Build history of the part. All positions in model axes, mm. Face numbers are marked on the shaded views. A direction names the side the tool comes from. Round coordinates to 2 decimals unless told otherwise and drop trailing zeros. Write each loop counter-clockwise with the first axis right and the second up, starting at its lowest first coordinate (ties: lowest second). Pieces come first, ordered by that corner, then holes. Notation, with made-up numbers: (34.25, 61.5) -> (45.25, 61.5) arc R19 ccw to (45.25, 95.5) -> close; hole circle Ø4 at (-13, -39.75). An arc over 180 degrees is marked (long way). One line per question, with ' | ' between items.
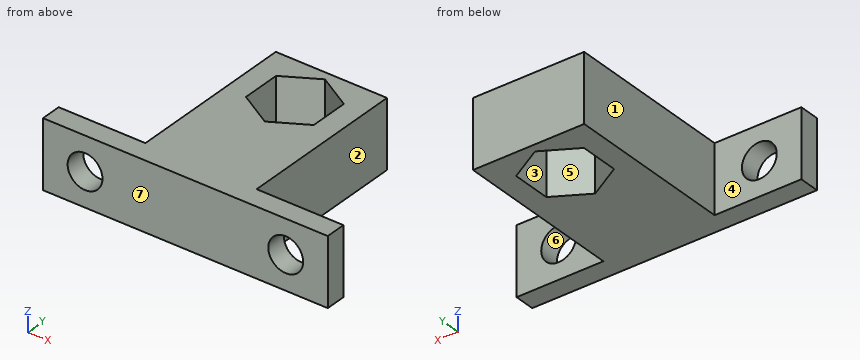
from build123d import *

# Parameters (mm, degrees)
SKETCH1_W           = 15.494
SKETCH1_H           = 12.7
SKETCH1_R           = 3.2639
SKETCH1_W_2         = 22.352
BOSS_EXTRUDE3_DEPTH = 3.81
SKETCH3_W           = 20.828
SKETCH3_H           = 12.7
BOSS_EXTRUDE4_DEPTH = 31.75
CUT_EXTRUDE3_REACH  = 14.7


with BuildPart() as part:
    # Sketch1 → Boss-Extrude3 (new body)
    with BuildSketch(Plane(origin=(0, 0, 0), x_dir=(1, 0, 0), z_dir=(0, 1, 0))):
        with Locations((-27.634045528, -3.236090754)):
            Rectangle(SKETCH1_W, SKETCH1_H)
        with Locations((-27.507045528, -3.236090754)):
            Circle(SKETCH1_R, mode=Mode.SUBTRACT)
        with Locations((-8.711045528, -3.236090754)):
            Rectangle(SKETCH1_W_2, SKETCH1_H)
        with Locations((10.211954472, -3.236090754)):
            Rectangle(SKETCH1_W, SKETCH1_H)
        with Locations((10.084954472, -3.236090754)):
            Circle(SKETCH1_R, mode=Mode.SUBTRACT)
    extrude(amount=BOSS_EXTRUDE3_DEPTH)

    # Sketch3 → Boss-Extrude4 (add)
    with BuildSketch(Plane(origin=(0, 3.81, 0), x_dir=(1, 0, 0), z_dir=(0, 1, 0))):
        with Locations((-8.711045528, -3.236090754)):
            Rectangle(SKETCH3_W, SKETCH3_H)
    extrude(amount=BOSS_EXTRUDE4_DEPTH)

    # Sketch5 → Cut-Extrude3 (cut, up to next)
    with BuildSketch(Plane(origin=(0, 0, -3.113909246), x_dir=(-1, 0, 0), z_dir=(0, 0, -1)), mode=Mode.PRIVATE) as cut_extrude3_sk1:
        Polygon((8.711045528, 34.002348419), (2.361045528, 30.336174209), (2.361045528, 23.003825791), (8.711045528, 19.337651581), (15.061045528, 23.003825791), (15.061045528, 30.336174209), align=None)
    cut_extrude3_tool1 = extrude(cut_extrude3_sk1.sketch, amount=-CUT_EXTRUDE3_REACH, mode=Mode.PRIVATE) & part.part
    add(cut_extrude3_tool1.solids().sort_by_distance((-8.711046, 26.67, -3.113909))[0], mode=Mode.SUBTRACT)


solid = part.part
(1) Wall check: line 1 (X direction, y = 25, z = 0.75); line 2 (X direction, y = 34.5, z = 5); line 3 (Y direction, x = -5, z = 8.25). Give the ranges that are in metal, low to high. Write a range as from..to.
Calculated:
line 1: -19.13..-15.06, -2.36..1.7 | line 2: -19.13..1.7 | line 3: 0..21.48, 31.86..35.56
(2) Slice it at A-A (y = 25). Write the cut outline in (x, z), then the cut area to 3 significant figures.
Calculated:
outline: (-19.13, -3.11) -> (-15.06, -3.11) -> (-15.06, 9.59) -> (-19.13, 9.59) -> close; (-2.36, -3.11) -> (1.7, -3.11) -> (1.7, 9.59) -> (-2.36, 9.59) -> close | area: 103 mm2
(3) Slice it at C-C (x = -3). Write the cut outline in (y, z), then the cut area to 3 significant figures.
Calculated:
outline: (0, -3.11) -> (22.63, -3.11) -> (22.63, 9.59) -> (0, 9.59) -> close; (30.71, -3.11) -> (35.56, -3.11) -> (35.56, 9.59) -> (30.71, 9.59) -> close | area: 349 mm2
(4) Drop flat-ended pins along their axis: pin 1 (3 mm diameter, centred on y = 25, z = 0.5, fed in from -X); pin 2 (4 mm diameter, centred on x = 11, z = 5, fed in from +Y); pin 3 (3.5 mm diameter, centred on y = 26.5, z = 4, fed in from +X). Give the stop position or say it passes through.
Calculated:
pin 1: x = -19.13 | pin 2: y = 3.81 | pin 3: x = 1.7
(5) 3-axis set-ups, long thin cutter, end or side, ignore diameter. For the marked faces 1, 2 and 3: which of +Z, -Z, +X, -X, +Y, -Y reach the whole face in a straight line?
Calculated:
face 1: +Z, -Z, -X, +Y | face 2: +Z, -Z, +X, +Y | face 3: +Z, -Z
(6) Mould opens along Y. For the marked faces 4, 5, 6 and 7 say: pulls with the +Y half, pulls with the -Y half, needs draft (parallel to the pull), parting line crosses it, or undercut.
Calculated:
face 4: pulls with the +Y half | face 5: undercut | face 6: needs draft | face 7: pulls with the -Y half
(7) Slice it at B-B (z = 2.25). Write the cut outline in (x, y).
Calculated:
outline: (-35.38, 0) -> (-30.62, 0) -> (-30.62, 3.81) -> (-35.38, 3.81) -> close; (-24.4, 0) -> (6.97, 0) -> (6.97, 3.81) -> (1.7, 3.81) -> (1.7, 35.56) -> (-19.13, 35.56) -> (-19.13, 3.81) -> (-24.4, 3.81) -> close; (13.2, 0) -> (17.96, 0) -> (17.96, 3.81) -> (13.2, 3.81) -> close; hole (-15.06, 23) -> (-8.71, 19.34) -> (-2.36, 23) -> (-2.36, 30.34) -> (-8.71, 34) -> (-15.06, 30.34) -> close
(8) Slice it at D-D (z = -1.75). Write the cut outline in (x, y).
Calculated:
outline: (-35.38, 0) -> (17.96, 0) -> (17.96, 3.81) -> (1.7, 3.81) -> (1.7, 35.56) -> (-19.13, 35.56) -> (-19.13, 3.81) -> (-35.38, 3.81) -> close; hole (-15.06, 23) -> (-8.71, 19.34) -> (-2.36, 23) -> (-2.36, 30.34) -> (-8.71, 34) -> (-15.06, 30.34) -> close
